For this review, use the dimensioned drawing (mm, ordinates from the lowest corner) and the shaded views. A direction names the side the tool comes from. Coordinates: 2 decimals unless noted, no trailing zeros. Order: outer loops, then holes, each group sorted by start corner. A loop starts at its lowest first (then second) coordinate and runs counter-clockwise, first axis right, second up. Notation, with made-up numbers: (60.5, 7) -> (106.5, 7) arc R36 ccw to (106.5, 43) -> close; hole circle Ø3 at (-36, 86.5). An arc over 180 degrees is marked (long way). Return JSON: item names as keys, results as strings. Group by question number.
Item 1: Take a section at A-A (x = 11.9). Write out the cut boundary in (y, z), then the cut area to 3 significant figures.
Item 2: Take a section at B-B (z = 2.7). Write out the cut boundary in (x, y).
Item 3: Machinability: for the marked faces 1 and 2, which of the approach directions +Z, -Z, +X, -X, +Y, -Y give a long, thin tool a straight path to every point of the face, cutting with its end or side? Answer none if there is none.
Item 4: Take a section at D-D (y = 6.5). Write out the cut boundary in (x, z).
Item 5: Take a section at C-C (y = 11.9). Write out the cut boundary in (x, z).
Item 6: Insertion check: pin 1 (1 mm diameter, centred on x = 11.5, y = 6.5, fed in from +Z). The pin has a flat end and moves straight along its axis. Give the tip position at first contact, or say it passes through.
Item 7: Draft analysis for pull direction X (two halves, no side actions). For the marked faces 3, 4, 5 and 6, state which applies: +X half, -X half, draft (parallel to the pull), parting line (faces both ways), or undercut.
Item 8: For line 1 along Z through (x, y) = (6.75, 6); line 2 along Y through (x, z) = (4, 2.9); line 3 along X through (y, z) = (9.75, 2.05), list the stretches that pass through material, from the lowest coordinate up.
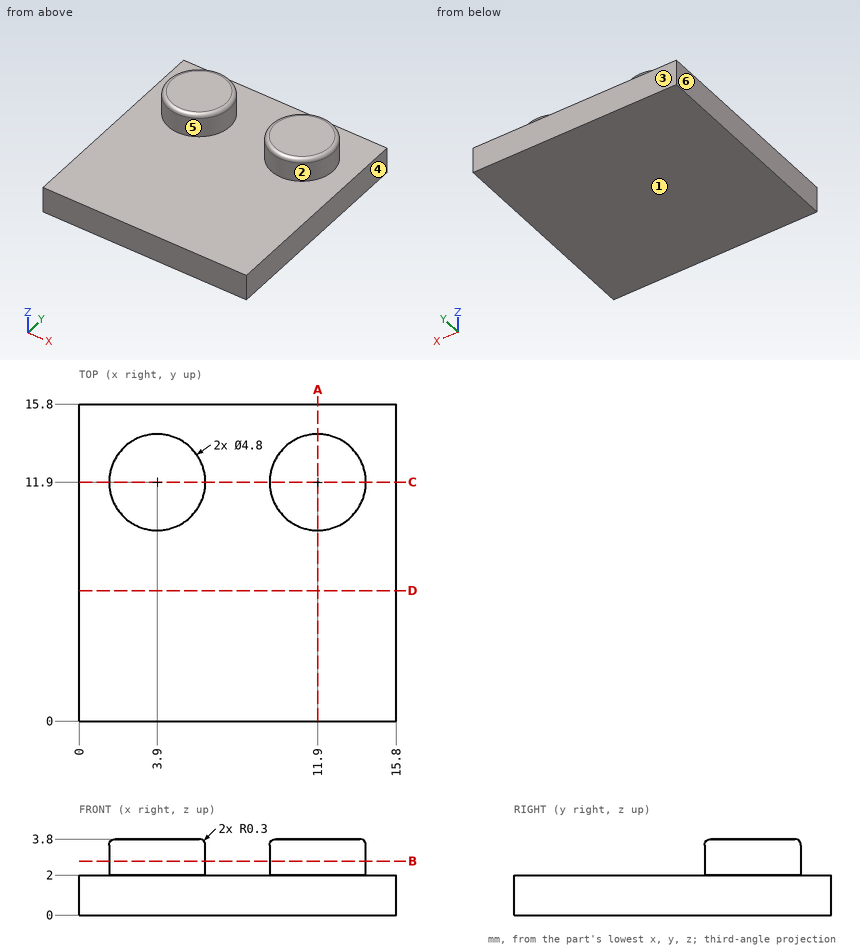
Findings below:
{
 "1": {"outline": "(0, 0) -> (15.8, 0) -> (15.8, 2) -> (14.3, 2) -> (14.3, 3.5) arc R0.3 ccw to (14, 3.8) -> (9.8, 3.8) arc R0.3 ccw to (9.5, 3.5) -> (9.5, 2) -> (0, 2) -> close", "area": "40.2 mm2"},
 "2": {"outline": "circle Ø4.8 at (3.9, 11.9); circle Ø4.8 at (11.9, 11.9)"},
 "3": {"face 1": "-Z, +X, -X, +Y, -Y", "face 2": "+Z"},
 "4": {"outline": "(0, 0) -> (15.8, 0) -> (15.8, 2) -> (0, 2) -> close"},
 "5": {"outline": "(0, 0) -> (15.8, 0) -> (15.8, 2) -> (14.3, 2) -> (14.3, 3.5) arc R0.3 ccw to (14, 3.8) -> (9.8, 3.8) arc R0.3 ccw to (9.5, 3.5) -> (9.5, 2) -> (6.3, 2) -> (6.3, 3.5) arc R0.3 ccw to (6, 3.8) -> (1.8, 3.8) arc R0.3 ccw to (1.5, 3.5) -> (1.5, 2) -> (0, 2) -> close"},
 "6": {"pin 1": "stops at z = 2"},
 "7": {"face 3": "draft", "face 4": "+X half", "face 5": "undercut", "face 6": "-X half"},
 "8": {"line 1": "z = 0 to 2", "line 2": "y = 9.5 to 14.3", "line 3": "x = 2.83 to 4.97, 10.83 to 12.97"}
}
